For this review, take the finished solid that the model builds, in its own axes (mm). Face numbers are marked on the shaded views. A direction names the side the tool comes from. Round coordinates to 2 decimals unless told otherwise and drop trailing zeros. Order: outer loops, then holes, each group sorted by start corner. A loop starts at its lowest first (then second) coordinate and runs counter-clockwise, first axis right, second up. Notation, with made-up numbers: M 20,-31 L 31,-31 A21 ccw 31,-7 Z; hole C -11.5,-33.75 d8. An arc over 180 degrees is marked long. Put each result on its own line as item: value.
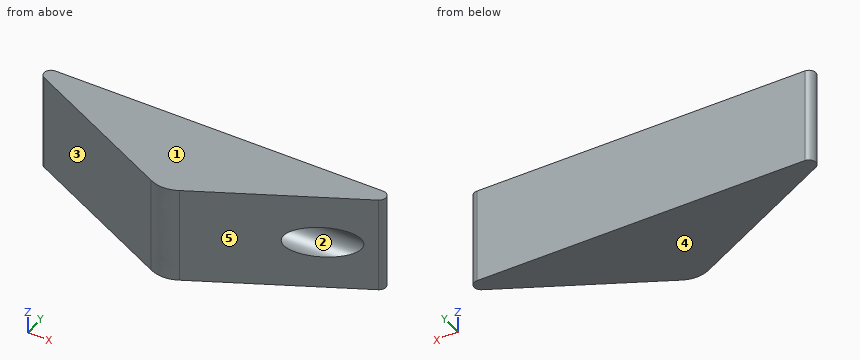
from build123d import *

# Parameters (mm, degrees)
F1_DEPTH    = 70
F2_R        = 5
F3_T1_DEPTH = 127.5
F5_D        = 23
F5_DEPTH    = 123.8206602125


# Not quite as in the source:
# - a fillet or chamfer that OpenCascade refuses, or shapes differently, is made with other operations: its cross-section is extruded or revolved along the edge and cut away or added


with BuildPart() as f1:
    # F0 (on Top) → F1 (new body)
    with BuildSketch(Plane.XY):
        Polygon((140, 70), (-140, 70), (0, 0), align=None)
    extrude(amount=F1_DEPTH)

    # F2
    f2_edges = [f1.edges().sort_by_distance(p)[0] for p in [
        (140, 70, 35),
        (-140, 70, 35),
    ]]
    fillet(f2_edges, radius=F2_R)

    # F3: fillet of radius 23 on 1 edges, made by hand

    # F3_s2 → F3_t1 (cut)
    with BuildSketch(Plane.XY.offset(-28.75)):
        with BuildLine():
            add(Edge.make_bspline(
                [(10.2859126965, 5.1429563482), (0, 0), (-10.2859126965, 5.1429563482)],
                knots=[0, 0, 0, 1, 1, 1], degree=2, weights=[1, 1, 1]))
            Line((-10.2859126965, 5.1429563482), (0, 0))
            Line((0, 0), (10.2859126965, 5.1429563482))
        make_face()
    extrude(amount=F3_T1_DEPTH, mode=Mode.SUBTRACT)

    # F5 (through all, one way)
    with BuildSketch(Plane(origin=(0, 0, 0), x_dir=(0, 1, 0), z_dir=(-1, 0, 0))):
        with Locations((45, -35)):
            Circle(F5_D / 2)
    extrude(amount=-F5_DEPTH, mode=Mode.SUBTRACT)


solid = f1.part
(1) Insertion check: pin 1 Ø18.5 at (y, z) = (48, 36) entering from +X; pin 2 Ø8 at (y, z) = (37.5, 42.5) entering from -X; pin 3 Ø1 at (y, z) = (45, 57) entering from +X. Each pin has a flat end and moves straight along its axis. Give the tip position at first contact, or say it passes through.
A:
pin 1: stops at x = 114.5
pin 2: stops at x = -83
pin 3: stops at x = 91
(2) Add section D-D on y = 7.5. Give the boundary of the cut face in (x, z).
A:
outline: M -15,0 L 15,0 L 15,70 L -15,70 Z
(3) For the marked faces 1 and 2, list the 3-axis set-ups (+Z, -Z, +X, -X, +Y, -Y) from which the entire face can be reached by the end or side of a thin tool; tool diameter is ignored.
A:
face 1: +Z, +X, -X, +Y, -Y
face 2: +X
(4) Add section C-C on x = -89.5. Give the boundary of the cut face in (y, z).
A:
outline: M 44.75,0 L 70,0 L 70,70 L 44.75,70 Z
(5) Draft analysis for pull direction X (two halves, no side actions). For the marked faces 3, 4 and 5, state which applies: released by +X, released by -X, zero draft, split by the parting line, or undercut.
A:
face 3: released by -X
face 4: zero draft
face 5: released by +X
(6) To check wall thickness, follow L1, parallel to Z at x = 28, y = 45; L2, parallel to Y at x = 77.5, z = 35; L3, parallel to Y at x = 27.5, z = 35. State the ranges of each line that lie inside material, in increasing order.
A:
L1: z = 0 to 23.5, 46.5 to 70
L2: y = 56.5 to 70
L3: y = 13.75 to 33.5, 56.5 to 70
(7) Add section A-A on x = 17. Give the boundary of the cut face in (y, z).
A:
outline: M 8.5,0 L 70,0 L 70,70 L 8.5,70 Z; hole C 45,35 d23
(8) Add section B-B on y = 45. Give the boundary of the cut face in (x, z), then the cut area to 3 significant figures.
A:
outline: M -90,0 L 90,0 L 90,23.5 L 0,23.5 L 0,46.5 L 90,46.5 L 90,70 L -90,70 Z
area: 10,500 mm2
